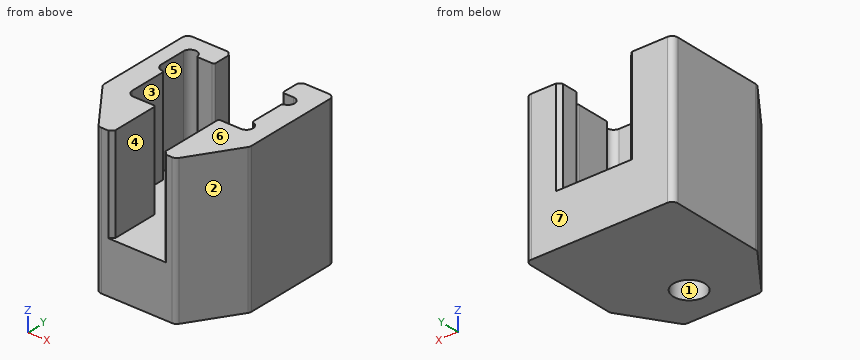
```python
from build123d import *

# Parameters (mm, degrees)
SALIENTE_EXTRUIR1_DEPTH                      = 38.5
CORTAR_EXTRUIR1_DEPTH                        = 25
REDONDEO2_R                                  = 0.5
REDONDEO3_R                                  = 1.5
PERFORADOR_PARA_ROSCAR_HELICOIL_DE_M81_D     = 8.25
PERFORADOR_PARA_ROSCAR_HELICOIL_DE_M81_DEPTH = 9.5
PERFORADOR_PARA_ROSCAR_HELICOIL_DE_M81_TIP   = 2.478550053
CHAFL_N1_SIZE                                = 1


with BuildPart() as part:
    # Croquis1 → Saliente-Extruir1 (new body)
    with BuildSketch(Plane.XY):
        Polygon((0, 13.3), (0, 39.7), (38.6, 39.7), (38.6, 13.3), (30.1, 0), (10, 0), align=None)
    extrude(amount=SALIENTE_EXTRUIR1_DEPTH)

    # Croquis2 → Cortar-Extruir1 (cut)
    with BuildSketch(Plane.XY.offset(38.5)):
        with BuildLine():
            Line((29.65, 39.7), (29.65, 34.1))
            Line((29.65, 34.1), (32.56, 34.1))
            ThreePointArc((32.56, 34.1), (34.31, 32.35), (32.56, 30.6))
            Line((32.56, 30.6), (32.56, 21.1))
            ThreePointArc((32.56, 21.1), (34.31, 19.35), (32.56, 17.6))
            Line((32.56, 17.6), (26.74, 17.6))
            Line((26.74, 17.6), (26.74, 0))
            Line((26.74, 0), (13.6, 0))
            Line((13.6, 0), (13.6, 13.65))
            Line((13.6, 13.65), (7.75, 13.65))
            ThreePointArc((7.75, 13.65), (6.512563133, 14.162563133), (6, 15.4))
            Line((6, 15.4), (6, 25.4))
            Line((6, 25.4), (5.5, 25.4))
            ThreePointArc((5.5, 25.4), (4.262563133, 25.912563133), (3.75, 27.15))
            Line((3.75, 27.15), (3.75, 34.1))
            ThreePointArc((3.75, 34.1), (5.5, 35.85), (7.25, 34.1))
            Line((7.25, 34.1), (11.79, 34.1))
            Line((11.79, 34.1), (11.79, 39.7))
            Line((11.79, 39.7), (29.65, 39.7))
        make_face()
    extrude(amount=-CORTAR_EXTRUIR1_DEPTH, mode=Mode.SUBTRACT)

    # Redondeo2
    redondeo2_edges = [part.edges().sort_by_distance(p)[0] for p in [
        (13.6, 13.65, 26),
        (11.79, 34.1, 26),
        (29.65, 34.1, 26),
        (32.56, 30.6, 26),
        (32.56, 21.1, 26),
        (26.74, 17.6, 26),
        (7.25, 34.1, 26),
        (6, 25.4, 26),
    ]]
    fillet(redondeo2_edges, radius=REDONDEO2_R - 0.0001)  # a hair under: the kernel refuses the full size

    # Redondeo3
    redondeo3_edges = [part.edges().sort_by_distance(p)[0] for p in [
        (0, 13.3, 19.25),
        (0, 39.7, 19.25),
        (38.6, 39.7, 19.25),
        (38.6, 13.3, 19.25),
        (30.1, 0, 19.25),
        (10, 0, 19.25),
    ]]
    fillet(redondeo3_edges, radius=REDONDEO3_R)

    # Perforador para roscar Helicoil de M81
    with Locations(Plane(origin=(0, 0, 0), x_dir=(-1, 0, 0), z_dir=(0, 0, -1))):
        with Locations((-20.6, 10)):
            Hole(PERFORADOR_PARA_ROSCAR_HELICOIL_DE_M81_D / 2, depth=PERFORADOR_PARA_ROSCAR_HELICOIL_DE_M81_DEPTH)
            with Locations((0, 0, -(PERFORADOR_PARA_ROSCAR_HELICOIL_DE_M81_DEPTH + PERFORADOR_PARA_ROSCAR_HELICOIL_DE_M81_TIP / 2))):  # 118° drill point
                Cone(0, PERFORADOR_PARA_ROSCAR_HELICOIL_DE_M81_D / 2, PERFORADOR_PARA_ROSCAR_HELICOIL_DE_M81_TIP, mode=Mode.SUBTRACT)

    # Chaflán1
    chafl_n1_edges = [part.edges().sort_by_distance(p)[0] for p in [
        (11.79, 39.7, 26),
        (29.65, 39.7, 26),
        (26.74, 0, 26),
        (13.6, 0, 26),
    ]]
    chamfer(chafl_n1_edges, length=CHAFL_N1_SIZE)


solid = part.part
```
For this review, take the finished solid that the model builds, in its own axes (mm). Face numbers are marked on the shaded views. A direction names the side the tool comes from. Coordinates: 2 decimals unless noted, no trailing zeros. Loops run counter-clockwise (first coordinate to the right, second up) from the corner with the lowest first, then second, coordinate; pieces in that order, holes last.
1. Insertion check: P1, Ø2.5, axis at x = 31.5, z = 20.5, coming from the -Y side; P2, Ø8, axis at y = 5.5, z = 32, coming from the -X side; P3, Ø10.5, axis at x = 20.6, y = 10, coming from the -Z side; P4, Ø5, axis at y = 8, z = 12.5, coming from the -X side. Each pin has a flat end and moves straight along its axis. Give the tip position at first contact, or say it passes through.
2. Add section A-A, the plane y = 28. Give the boundary of the cut face in (x, z), then the cut area to 3 significant figures.
3. Mouldability with a two-part tool opening along Y and no side actions: class the marked faces 5, 6 and 7 as +Y half, -Y half, draft (parallel to the pull), parting line (faces both ways), or undercut.
4. Add section D-D, the plane y = 19.5. Give the boundary of the cut face in (x, z).
5. Add section B-B, the plane z = 11. Give the boundary of the cut face in (x, y), then the cut area to 3 significant figures.
6. For line 1 (Y direction, x = 20.6, z = 7.25) (3 decimals); line 2 (Z direction, x = 7.5, y = 16.5); line 3 (X direction, y = 19.5, z = 21.5), list the stretches that pass through material, from the lowest coordinate up.
7. For the marked faces 1, 2, 3 and 4, list the 3-axis set-ups (+Z, -Z, +X, -X, +Y, -Y) from which the entire face can be reached by the end or side of a thin tool; tool diameter is ignored.
8. Add section C-C, the plane x = 25.5. Give the boundary of the cut face in (y, z).
Result:
1. P1: stops at y = 0.36
1. P2: stops at x = 2.86
1. P3: stops at z = 0
1. P4: stops at x = 2.11
2. outline: (0, 0) - (38.6, 0) - (38.6, 38.5) - (32.56, 38.5) - (32.56, 13.5) - (3.75, 13.5) - (3.75, 38.5) - (0, 38.5) - close
2. area: 766 mm2
3. face 5: undercut
3. face 6: draft
3. face 7: +Y half
4. outline: (0, 0) - (38.6, 0) - (38.6, 38.5) - (34.3, 38.5) - (34.3, 13.5) - (6, 13.5) - (6, 38.5) - (0, 38.5) - close
5. outline: (0, 13.8) arc R1.5 ccw to (0.3, 12.9) - (9.55, 0.6) arc R1.5 ccw to (10.75, 0) - (29.28, 0) arc R1.5 ccw to (30.54, 0.69) - (38.36, 12.93) arc R1.5 ccw to (38.6, 13.74) - (38.6, 38.2) arc R1.5 ccw to (37.1, 39.7) - (1.5, 39.7) arc R1.5 ccw to (0, 38.2) - close; hole circle Ø3.26 at (20.6, 10)
5. area: 1,400 mm2
6. line 1: y = 0 to 5.875, 14.125 to 39.7
6. line 2: z = 0 to 13.5
6. line 3: x = 0 to 6, 34.3 to 38.6
7. face 1: -Z
7. face 2: +Z, -Z, +X, -Y
7. face 3: +Z
7. face 4: +Z, +Y, -Y
8. outline: (0, 0) - (39.7, 0) - (39.7, 13.5) - (0, 13.5) - close
